Design review of the part built by this model. Coordinates are the model's own, in mm. Face numbers are marked on the shaded views. A direction names the side the tool comes from. Give positions to 0.01 mm unless a question says otherwise; leave off trailing zeros. Write each loop counter-clockwise with the first axis right and the second up, starting at its lowest first coordinate (ties: lowest second). Pieces come first, ordered by that corner, then holes.
```python
from build123d import *

# Parameters (mm, degrees)
SKETCH_2_W               = 90
SKETCH_2_H               = 89
EXTRUDE_1_DEPTH          = 13
SKETCH_3_W               = 89
SKETCH_3_H               = 58
EXTRUDE_2_DEPTH          = 13
FILLET_1_R               = 25
EXTRUDE_4_DEPTH          = 13
SKETCH_5_R               = 12.5
CUT_EXTRUDE_1_DEPTH      = 134.792817279
FILLET_2_R               = 25
CUT_EXTRUDE_2_DEPTH      = 152.201803843
SKETCH_7_R               = 38
EXTRUDE_5_DEPTH          = 13
CUT_EXTRUDE_3_DEPTH      = 13
CUT_EXTRUDE_3_DEPTH_BACK = 19
SKETCH_7_3_R             = 28.5
EXTRUDE_START            = -13
SKETCH_7_4_R             = 28.5
EXTRUDE_6_DEPTH          = 21
SKETCH_7_5_R             = 12.5
CUT_EXTRUDE_4_DEPTH      = 120.960410109
SKETCH_8_W               = 11.780980298
SKETCH_8_H               = 3.266568958
CUT_EXTRUDE_5_DEPTH      = 21
EXTRUDE_7_DEPTH          = 89
EXTRUDE_START_2          = -21
SKETCH_7_6_R             = 38
EXTRUDE_8_DEPTH          = 21
SKETCH_7_7_R             = 28.5
CUT_EXTRUDE_6_DEPTH      = 15


with BuildPart() as part:
    # Sketch 2 → Extrude 1 (new body)
    with BuildSketch(Plane(origin=(0, 0, 0), x_dir=(1, 0, 0), z_dir=(0, 1, 0))):
        Rectangle(SKETCH_2_W, SKETCH_2_H)
    extrude(amount=EXTRUDE_1_DEPTH)

    # Sketch 3 → Extrude 2 (add)
    with BuildSketch(Plane(origin=(29, 29, 0), x_dir=(0, 0, -1), z_dir=(-0.7071067811865438, -0.7071067811865512, 0))):
        with Locations((0, 51.627416998)):
            Rectangle(SKETCH_3_W, SKETCH_3_H)
    extrude(amount=EXTRUDE_2_DEPTH)

    # Fillet 1
    fillet_1_edges = [part.edges().sort_by_distance(p)[0] for p in [
        (81.415999231, -32.608387387, 44.5),
        (81.415999231, -32.608387387, -44.5),
    ]]
    fillet(fillet_1_edges, radius=FILLET_1_R)

    # Sketch 4 → Extrude 4 (add)
    with BuildSketch(Plane(origin=(-16, -16, 0), x_dir=(0, 0, -1), z_dir=(-0.7071067811865438, -0.7071067811865512, 0))):
        Polygon((44.5, -105.012193309), (44.5, -41.012193309), (44.5, -36.415999231), (-44.5, -36.415999231), (-44.5, -41.012193309), (-44.5, -105.012193309), align=None)
    extrude(amount=EXTRUDE_4_DEPTH)

    # Sketch 5 → Cut-Extrude 1 (cut, through all)
    with BuildSketch(Plane(origin=(-16, -16, 0), x_dir=(0, 0, -1), z_dir=(0.707106781186544, 0.7071067811865511, 0))):
        with Locations(Location((-19, 85.012193309, 0), (0, 0, 90))):
            Circle(SKETCH_5_R)
        with Locations(Location((18.938317585, 82.847924647, 0), (0, 0, 90))):
            Circle(SKETCH_5_R)
    extrude(amount=-CUT_EXTRUDE_1_DEPTH, mode=Mode.SUBTRACT)

    # Fillet 2
    fillet_2_edges = [part.edges().sort_by_distance(p)[0] for p in [
        (-94.851028074, 53.658639918, -44.5),
        (-94.851028074, 53.658639918, 44.5),
    ]]
    fillet(fillet_2_edges, radius=FILLET_2_R)

    # Sketch 6 → Cut-Extrude 2 (cut, through all)
    with BuildSketch(Plane(origin=(29, 29, 0), x_dir=(0, 0, -1), z_dir=(0.707106781186544, 0.7071067811865511, 0))):
        with BuildLine():
            Line((-18.50653718, -48.627416998), (19.49346282, -48.627416998))
            ThreePointArc((19.49346282, -48.627416998), (29.49346282, -58.627416998), (19.49346282, -68.627416998))
            Line((19.49346282, -68.627416998), (-18.50653718, -68.627416998))
            ThreePointArc((-18.50653718, -68.627416998), (-28.50653718, -58.627416998), (-18.50653718, -48.627416998))
        make_face()
    extrude(amount=-CUT_EXTRUDE_2_DEPTH, mode=Mode.SUBTRACT)

    # Sketch 7 → Extrude 5 (add)
    with BuildSketch(Plane(origin=(0, 13, 0), x_dir=(1, 0, 0), z_dir=(0, 1, 0))):
        with Locations(Location((0, 0, 0), (0, 0, 90))):
            Circle(SKETCH_7_R)
    extrude(amount=EXTRUDE_5_DEPTH)

    # Sketch 7_3 → Cut-Extrude 3 (cut, two sides: drawn at the far end of the back side and taken through both)
    with BuildSketch(Plane(origin=(0, 13, 0), x_dir=(1, 0, 0), z_dir=(0, 1, 0)).offset(-CUT_EXTRUDE_3_DEPTH_BACK)):
        with Locations(Location((0, 0, 0), (0, 0, 270))):
            Circle(SKETCH_7_3_R)
    extrude(amount=CUT_EXTRUDE_3_DEPTH + CUT_EXTRUDE_3_DEPTH_BACK, mode=Mode.SUBTRACT)

    # Sketch 8 → Cut-Extrude 5 (cut)
    with BuildSketch(Plane(origin=(0, 13, 0), x_dir=(1, 0, 0), z_dir=(0, 1, 0))):
        with Locations((-2.280738609, 42.866715521)):
            Rectangle(SKETCH_8_W, SKETCH_8_H)
        with Locations((-2.280738609, -42.866715521)):
            Rectangle(SKETCH_8_W, SKETCH_8_H)
    extrude(amount=-CUT_EXTRUDE_5_DEPTH, mode=Mode.SUBTRACT)

    # Sketch 9 → Extrude 7 (add)
    with BuildSketch(Plane(origin=(0, 0, -44.5), x_dir=(-1, 0, 0), z_dir=(0, 0, -1))):
        Polygon((45, 6.5), (45, 0), (50.942388155, 0.557611845), align=None)
    extrude(amount=-EXTRUDE_7_DEPTH)



with BuildPart() as body_2:
    # Sketch 7_4 → Extrude 6 (new body)
    with BuildSketch(Plane(origin=(0, 13, 0), x_dir=(1, 0, 0), z_dir=(0, 1, 0)).offset(EXTRUDE_START)):
        with Locations(Location((0, 0, 0), (0, 0, 270))):
            Circle(SKETCH_7_4_R)
    extrude(amount=-EXTRUDE_6_DEPTH)

    # Sketch 7_5 → Cut-Extrude 4 (cut, through all)
    with BuildSketch(Plane(origin=(0, 13, 0), x_dir=(1, 0, 0), z_dir=(0, 1, 0))):
        with Locations(Location((0, 0, 0), (0, 0, 270))):
            Circle(SKETCH_7_5_R)
    extrude(amount=-CUT_EXTRUDE_4_DEPTH, mode=Mode.SUBTRACT)


with BuildPart() as part_1:
    add(part.part)

    add(body_2.part)  # Extrude 8 merges body 2
    # Sketch 7_6 → Extrude 8 (add)
    with BuildSketch(Plane(origin=(0, 13, 0), x_dir=(1, 0, 0), z_dir=(0, 1, 0)).offset(EXTRUDE_START_2)):
        with Locations(Location((0, 0, 0), (0, 0, 270))):
            Circle(SKETCH_7_6_R)
    extrude(amount=EXTRUDE_8_DEPTH)

    # Sketch 7_7 → Cut-Extrude 6 (cut)
    with BuildSketch(Plane(origin=(0, 13, 0), x_dir=(1, 0, 0), z_dir=(0, 1, 0))):
        with Locations(Location((0, 0, 0), (0, 0, 270))):
            Circle(SKETCH_7_7_R)
    extrude(amount=-CUT_EXTRUDE_6_DEPTH, mode=Mode.SUBTRACT)


solid = part_1.part
```
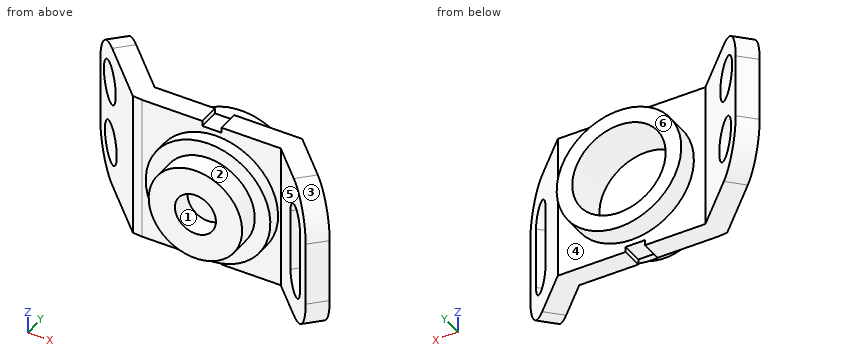
(1) Clearance check with flat-ended pins moving along their axes: P1, Ø8, axis at x = -50.5, z = 22, coming from the -Y side; P2, Ø1.5, axis at x = 15.5, z = 28.5, coming from the +Y side; P3, Ø2.5, axis at y = 7, z = 42, coming from the +X side. State where each tip first meets the part, or that it passes through.
Resolved:
P1: stops at y = 0.14
P2: stops at y = 26
P3: stops at x = 52.25
(2) Consider section A-A, the plane x = 0. Give the boundary of the cut face in (y, z).
Resolved:
outline: (-21, -28.5) - (-8, -28.5) - (-8, -38) - (0, -38) - (0, -41.23) - (13, -41.23) - (13, -38) - (26, -38) - (26, -28.5) - (-2, -28.5) - (-2, 28.5) - (26, 28.5) - (26, 38) - (13, 38) - (13, 41.23) - (0, 41.23) - (0, 38) - (-8, 38) - (-8, 28.5) - (-21, 28.5) - (-21, 12.5) - (-8, 12.5) - (-8, -12.5) - (-21, -12.5) - close
(3) Consider section C-C, the plane y = 10. Give the boundary of the cut face in (x, z).
Resolved:
outline: (-60.38, -44.5) - (-8.17, -44.5) - (-8.17, -41.23) - (3.61, -41.23) - (3.61, -44.5) - (48, -44.5) - (48, 44.5) - (3.61, 44.5) - (3.61, 41.23) - (-8.17, 41.23) - (-8.17, 44.5) - (-60.38, 44.5) - close; hole circle Ø57 at (0, 0)
(4) Consider section D-D, the plane x = 33. Give the boundary of the cut face in (y, z), then the cut area to 3 significant figures.
Resolved:
outline: (-8, -18.84) - (0, -18.84) - (0, -44.5) - (13, -44.5) - (13, -18.84) - (26, -18.84) - (26, 18.84) - (13, 18.84) - (13, 44.5) - (0, 44.5) - (0, 18.84) - (-8, 18.84) - close
area: 1,950 mm2
(5) Tool access review of the marked faces 4, 5 and 6: name each direction out of +Z, -Z, +X, -X, +Y, -Y from which nothing blocks a thin tool from reaching the whole face with its end or side.
Resolved:
face 4: +Y
face 5: +Z, -Z, -Y
face 6: +Z, -Z, +X, +Y
(6) To check wall thickness, follow L1, parallel to X at y = -11, z = 0; L2, parallel to X at y = 15, z = 0; L3, parallel to Y at x = 6, z = 23.5. State the ranges of each line that lie inside material, in increasing order.
Resolved:
L1: x = -28.5 to -12.5, 12.5 to 28.5, 50.62 to 57.77
L2: x = -65.38 to -47, -38 to -28.5, 28.5 to 38
L3: y = -21 to -2
(7) Mouldability with a two-part tool opening along Z and no side actions: class the marked faces 1, 2 and 3 as pulls with the +Z half, pulls with the -Z half, needs draft (parallel to the pull), parting line crosses it, or undercut.
Resolved:
face 1: undercut
face 2: parting line crosses it
face 3: pulls with the +Z half
